Part model, mm, in its own coordinate system. Face numbers are marked on the shaded views. A direction names the side the tool comes from. Give positions to 0.01 mm unless a question says otherwise; leave off trailing zeros. Order: outer loops, then holes, each group sorted by start corner. A loop starts at its lowest first (then second) coordinate and runs counter-clockwise, first axis right, second up. Notation, with made-up numbers: (84, -4.5) - (111, -4.5) arc R20 ccw to (111, 29.5) - close; hole circle Ø2 at (7.5, 12.25). An arc over 180 degrees is marked (long way). Use a Markdown table: item, result. Add a question column.
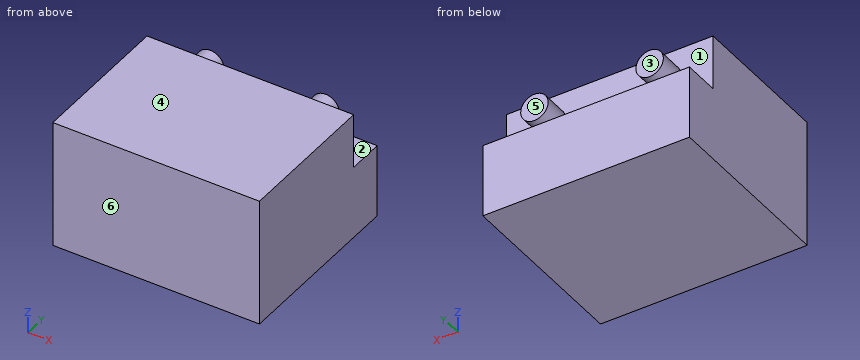
from build123d import *

# Parameters (mm, degrees)
SKETCH1_W           = 113
SKETCH1_H           = 70
BOSS_EXTRUDE1_DEPTH = 100
SKETCH2_W           = 113
SKETCH2_H           = 30
CUT_EXTRUDE2_DEPTH  = 20
SKETCH3_R           = 7.5
BOSS_EXTRUDE2_DEPTH = 15


with BuildPart() as part:
    # Sketch1 → Boss-Extrude1 (new body)
    with BuildSketch(Plane(origin=(0, 0, 0), x_dir=(1, 0, 0), z_dir=(0, 1, 0))):
        Rectangle(SKETCH1_W, SKETCH1_H)
    extrude(amount=BOSS_EXTRUDE1_DEPTH)

    # Sketch2 → Cut-Extrude2 (cut)
    with BuildSketch(Plane(origin=(0, 100, 0), x_dir=(1, 0, 0), z_dir=(0, 1, 0))):
        with Locations((0, -20)):
            Rectangle(SKETCH2_W, SKETCH2_H)
    extrude(amount=-CUT_EXTRUDE2_DEPTH, mode=Mode.SUBTRACT)

    # Sketch3 → Boss-Extrude2 (add)
    with BuildSketch(Plane(origin=(0, 80, 0), x_dir=(1, 0, 0), z_dir=(0, 1, 0))):
        with Locations((-31.5, -20)):
            Circle(SKETCH3_R)
        with Locations((31.5, -20)):
            Circle(SKETCH3_R)
    extrude(amount=BOSS_EXTRUDE2_DEPTH)


solid = part.part
1. Tool access for the marked faces 1, 2 and 3: list every direction of +Z, -Z, +X, -X, +Y, -Y with a clear straight run to the whole face (end or side of a thin tool).
2. Pin check, flat tips, straight feed: P1, Ø1, axis at x = 15, z = 10, coming from the +Y side; P2, Ø4.5, axis at x = -33.5, z = 20.5, coming from the +Y side; P3, Ø22, axis at x = -8, y = 92, coming from the +Z side. Stop position of each tip, or through.
3. Cut at C-C (x = -44). Write the cut outline in (y, z), plus the area to 3 significant figures.
4. Cut at A-A (z = 24.5). Write the cut outline in (x, y).
5. Drill centre lines: probe 1 along Y at (x, z) = (41, 16); probe 2 along Z at (x, y) = (50.5, 88.5); probe 3 along Y at (x, z) = (-28, 19). Where is each one in solid material? Low to high. Write a range as [from, to].
6. Cut at D-D (z = 8). Write the cut outline in (x, y), plus the area to 3 significant figures.
7. Mould opens along Y. For the marked faces 4, 5 and 6 say: released by +Y, released by -Y, zero draft, split by the parting line, or undercut.
8. Cut at B-B (x = -31.5). Write the cut outline in (y, z).
Responses:
| question | item | result |
|---|---|---|
| 1 | face 1 | +Y |
| 1 | face 2 | +X, -X, +Y |
| 1 | face 3 | +Z, +X, -X, +Y |
| 2 | P1 | stops at y = 80 |
| 2 | P2 | stops at y = 95 |
| 2 | P3 | stops at z = 5 |
| 3 | outline | (0, -35) - (100, -35) - (100, 5) - (80, 5) - (80, 35) - (0, 35) - close |
| 3 | area | 6,400 mm² |
| 4 | outline | (-56.5, 0) - (56.5, 0) - (56.5, 80) - (37.5, 80) - (37.5, 95) - (25.5, 95) - (25.5, 80) - (-25.5, 80) - (-25.5, 95) - (-37.5, 95) - (-37.5, 80) - (-56.5, 80) - close |
| 5 | probe 1 | y = [0, 80] |
| 5 | probe 2 | z = [-35, 5] |
| 5 | probe 3 | y = [0, 95] |
| 6 | outline | (-56.5, 0) - (56.5, 0) - (56.5, 80) - (-56.5, 80) - close |
| 6 | area | 9,040 mm² |
| 7 | face 4 | zero draft |
| 7 | face 5 | released by +Y |
| 7 | face 6 | released by -Y |
| 8 | outline | (0, -35) - (100, -35) - (100, 5) - (80, 5) - (80, 12.5) - (95, 12.5) - (95, 27.5) - (80, 27.5) - (80, 35) - (0, 35) - close |
